Can you work these out from the model? Positions are in its coordinate system, mm. Coordinates: 2 decimals unless noted, no trailing zeros. Order: outer loops, then holes, each group sorted by start corner. A loop starts at its lowest first (then second) coordinate and runs counter-clockwise, first axis right, second up. Notation, with made-up numbers: M 76,54.25 L 86,54.25 A22 ccw 86,90.25 Z; hole C 68,-16 d10. An arc over 180 degrees is marked long. Answer as CSV lines item,"result". Start each with the question number.
1. I need wall thicknesses on line 1 along X through (y, z) = (9, 3); line 2 along Y through (x, z) = (-0.5, 2); line 3 along X through (y, z) = (15.5, 4). Which ranges of each line are inside material? Lowest first, please. Write a range as from..to.
2. If we section it at B-B (x = -7): List the corners of the cut face in (y, z) for me.
3. If we section it at D-D (z = 1): Give the number of separate pieces and of enclosed holes in the cut face, plus the area to 3 significant figures.
4. If we section it at C-C (y = 13): List the corners of the cut face in (x, z) for me, plus the area to 3 significant figures.
5. Will these pins go through, and if not, where does the flat tip stop? pin 1 (2 mm diameter, centred on y = 19.5, z = 5.5, fed in from +X); pin 2 (6 mm diameter, centred on x = 10, z = 6, fed in from -Y); pin 3 (2 mm diameter, centred on y = -20.5, z = 1, fed in from -X).
6. If we mould it in two halves opening along Y, with no side actions, what happens to faces 1 (the face through (24.63, 17.13, 4.93)), 2 (the face through (-1.5, 0, 5)), 3 (the face through (0, -2, 0)), 4 (the face through (0, -29, 5))? For each: released by +Y, released by -Y, zero draft, split by the parting line, or undercut.
7. If we section it at A-A (y = -12.5): List the corners of the cut face in (x, z) for me.
```python
from build123d import *

# Parameters (mm, degrees)
SKETCH_W  = 3
SKETCH_H  = 3
PAD_DEPTH = 10


with BuildPart() as part:
    # Sketch → Pad (new body)
    with BuildSketch(Plane.XY):
        with BuildLine():
            ThreePointArc((29.690766, -4.296324), (29.885841, 2.614672), (28.493648, 9.3868))
            ThreePointArc((28.493648, 9.3868), (28.425702, 10.346109), (27.86112, 11.124658))
            ThreePointArc((27.86112, 11.124658), (24.574561, 17.207293), (19.982823, 22.376032))
            ThreePointArc((19.982823, 22.376032), (19.444325, 23.172844), (18.566109, 23.564796))
            ThreePointArc((18.566109, 23.564796), (12.678548, 27.189234), (6.117616, 29.369623))
            ThreePointArc((6.117616, 29.369623), (5.252857, 29.790435), (4.296324, 29.690766))
            ThreePointArc((4.296324, 29.690766), (-2.614672, 29.885841), (-9.3868, 28.493648))
            ThreePointArc((-9.3868, 28.493648), (-10.346109, 28.425702), (-11.124658, 27.86112))
            ThreePointArc((-11.124658, 27.86112), (-17.207293, 24.574561), (-22.376032, 19.982823))
            ThreePointArc((-22.376032, 19.982823), (-23.172844, 19.444325), (-23.564796, 18.566109))
            ThreePointArc((-23.564796, 18.566109), (-27.189234, 12.678548), (-29.369623, 6.117616))
            ThreePointArc((-29.369623, 6.117616), (-29.790435, 5.252857), (-29.690766, 4.296324))
            ThreePointArc((-29.690766, 4.296324), (-29.885841, -2.614672), (-28.493648, -9.3868))
            ThreePointArc((-28.493648, -9.3868), (-28.425702, -10.346109), (-27.86112, -11.124658))
            ThreePointArc((-27.86112, -11.124658), (-24.574561, -17.207293), (-19.982823, -22.376032))
            ThreePointArc((-19.982823, -22.376032), (-19.444325, -23.172844), (-18.566109, -23.564796))
            ThreePointArc((-18.566109, -23.564796), (-12.678548, -27.189234), (-6.117616, -29.369623))
            ThreePointArc((-6.117616, -29.369623), (-5.252857, -29.790435), (-4.296324, -29.690766))
            ThreePointArc((-4.296324, -29.690766), (2.614672, -29.885841), (9.3868, -28.493648))
            ThreePointArc((9.3868, -28.493648), (10.346109, -28.425702), (11.124658, -27.86112))
            ThreePointArc((11.124658, -27.86112), (17.552516, -24.329184), (22.931281, -19.343122))
            ThreePointArc((22.931281, -19.343122), (22.98258, -19.284674), (23.031232, -19.224005))
            ThreePointArc((23.031232, -19.224005), (27.007531, -13.061135), (29.369623, -6.117616))
            ThreePointArc((29.369623, -6.117616), (29.790435, -5.252857), (29.690766, -4.296324))
        make_face()
        with BuildLine():
            ThreePointArc((27.238634, -9.95273), (25.114737, 14.5), (5, 28.565714))
            Line((5, 28.565714), (2, 5.656854))
            ThreePointArc((5.898979, -1.096376), (5.196152, 3), (2, 5.656854))
            Line((5.898979, -1.096376), (27.238634, -9.95273))
        make_face(mode=Mode.SUBTRACT)
        with BuildLine():
            ThreePointArc((-22.238634, -18.612984), (0, -29), (22.238634, -18.612984))
            Line((3.898979, -4.560478), (22.238634, -18.612984))
            ThreePointArc((-3.898979, -4.560478), (0, -6), (3.898979, -4.560478))
            Line((-3.898979, -4.560478), (-22.238634, -18.612984))
        make_face(mode=Mode.SUBTRACT)
        with BuildLine():
            ThreePointArc((-5, 28.565714), (-25.114737, 14.5), (-27.238634, -9.95273))
            Line((-5.898979, -1.096376), (-27.238634, -9.95273))
            ThreePointArc((-2, 5.656854), (-5.196152, 3), (-5.898979, -1.096376))
            Line((-5, 28.565714), (-2, 5.656854))
        make_face(mode=Mode.SUBTRACT)
        Rectangle(SKETCH_W, SKETCH_H, mode=Mode.SUBTRACT)
    extrude(amount=PAD_DEPTH)


solid = part.part
```
Solved:
1,line 1,"-28.62..-27.57, -2.44..2.44, 27.57..28.62"
1,line 2,"-30..-29, -5.98..-1.5, 1.5..30"
1,line 3,"-25.69..-24.51, -3.29..3.29, 24.51..25.69"
2,outline,"M -29.17,0 L -28.14,0 L -28.14,10 L -29.17,10 Z; M -6.94,0 L -1.55,0 L -1.55,10 L -6.94,10 Z; M 28.14,0 L 29.17,0 L 29.17,10 L 28.14,10 Z"
3,separate pieces,"1"
3,enclosed holes,"4"
3,area,"780 mm²"
4,outline,"M -27.04,0 L -25.92,0 L -25.92,10 L -27.04,10 Z; M -2.96,0 L 2.96,0 L 2.96,10 L -2.96,10 Z; M 25.92,0 L 27.04,0 L 27.04,10 L 25.92,10 Z"
4,area,"81.5 mm²"
5,pin 1,"x = 23.62"
5,pin 2,"y = -29.17"
5,pin 3,"x = -22.8"
6,face 1,"released by +Y"
6,face 2,"undercut"
6,face 3,"zero draft"
6,face 4,"undercut"
7,outline,"M -27.27,0 L -14.26,0 L -14.26,10 L -27.27,10 Z; M 14.26,0 L 27.27,0 L 27.27,10 L 14.26,10 Z"
